Input: part model. Units: mm. Frame: model coordinates. A direction names the side the tool comes from. Coordinates: 2 decimals unless noted, no trailing zeros. Order: outer loops, then holes, each group sorted by start corner. A loop starts at its lowest first (then second) coordinate and runs counter-clockwise, first axis right, second up. Notation, with made-up numbers: (31.5, 54) -> (51.5, 54) arc R22 cw to (51.5, 84) -> close; hole circle Ø10 at (24.25, 70.25). An arc over 180 degrees is marked (long way). One line per question, with ' | ' between items.
```python
from build123d import *

# Parameters (mm, degrees)
F0_W     = 19.05
F0_H     = 19.05
F1_DEPTH = 9.525
F2_R     = 6.35
F3_DEPTH = 12.7
F4_R     = 9.525
F4_R_2   = 6.35
F5_DEPTH = 12.7


with BuildPart() as f1:
    # F0 (on Top) → F1 (new body, symmetric)
    with BuildSketch(Plane.XY):
        Rectangle(F0_W, F0_H)
    extrude(amount=F1_DEPTH, both=True)

    # F2 (on face) → F3 (join)
    with BuildSketch(Plane(origin=(0, 9.525, 0), x_dir=(-1, 0, 0), z_dir=(0, 1, 0))):
        with BuildLine():
            ThreePointArc((0, -9.525), (6.7351920908, -6.7351920908), (9.525, 0))
            ThreePointArc((9.525, 0), (6.7351920908, 6.7351920908), (0, 9.525))
            ThreePointArc((0, 9.525), (-6.7351920908, 6.7351920908), (-9.525, 0))
            ThreePointArc((-9.525, 0), (-6.7351920908, -6.7351920908), (0, -9.525))
        make_face()
        Circle(F2_R, mode=Mode.SUBTRACT)
    extrude(amount=F3_DEPTH)

    # F4 (on face) → F5 (join)
    with BuildSketch(Plane(origin=(-9.525, 0, 0), x_dir=(0, -1, 0), z_dir=(-1, 0, 0))):
        Circle(F4_R)
        Circle(F4_R_2, mode=Mode.SUBTRACT)
    extrude(amount=F5_DEPTH)


solid = f1.part
```
1. Cut plane D-D, the plane y = -5. Return loops of the section in (x, z) (3 decimals).
Recorded:
outline: (-22.225, -8.107) -> (-9.525, -8.107) -> (-9.525, -9.525) -> (9.525, -9.525) -> (9.525, 9.525) -> (-9.525, 9.525) -> (-9.525, 8.107) -> (-22.225, 8.107) -> (-22.225, 3.914) -> (-9.525, 3.914) -> (-9.525, -3.914) -> (-22.225, -3.914) -> close
2. Mould query, pull axis Y, two halves, no side actions, for faces 1 (the face through (-9.525, -8, -7)), 2 (the face through (-15.79, 1.38, -6.2)), 3 (the face through (-6.2, 22.225, -2)), 4 (the face through (-9.525, 0, 0)). Classes: released by +Y, released by -Y, zero draft, split by the parting line, or undercut.
Recorded:
face 1: zero draft | face 2: undercut | face 3: released by +Y | face 4: undercut
3. Cut plane B-B, the plane z = -4. Return loops of the section in (x, y) (3 decimals), and give its area (3 significant figures).
Recorded:
outline: (-22.225, -8.644) -> (-9.525, -8.644) -> (-9.525, -9.525) -> (9.525, -9.525) -> (9.525, 9.525) -> (8.644, 9.525) -> (8.644, 22.225) -> (4.932, 22.225) -> (4.932, 9.525) -> (-4.932, 9.525) -> (-4.932, 22.225) -> (-8.644, 22.225) -> (-8.644, 9.525) -> (-9.525, 9.525) -> (-9.525, 8.644) -> (-22.225, 8.644) -> (-22.225, 4.932) -> (-9.525, 4.932) -> (-9.525, -4.932) -> (-22.225, -4.932) -> close | area: 552 mm^2
4. Access query for faces 5 (the face through (0, 9.525, 0)), 6 (the face through (-15.786, 7.559, -5.796)), 7 (the face through (-8, 9.525, 7)), 8 (the face through (-9.525, 8, -8)), 9 (the face through (8, 9.525, -8)). Directions: +Z, -Z, +X, -X, +Y, -Y. A direction counts if a zero-diameter tool reaches every point of the face in a straight line with its end or side. Return the directions, or none.
Recorded:
face 5: +Y | face 6: -X | face 7: +Z, -X, +Y | face 8: -Z, -X, +Y | face 9: -Z, +X, +Y
5. Cut plane A-A, the plane x = -19. Return loops of the section in (y, z) (3 decimals).
Recorded:
outline: circle Ø19.05 at (0, 0); hole circle Ø12.7 at (0, 0)
6. Ray query, line 1 (Z direction, x = -12, y = 0) (3 decimals); line 2 (Y direction, x = 0, z = -3.5) (3 decimals). Return the intervals inside material, ascending. Write a range as [from, to].
Recorded:
line 1: z = [-9.525, -6.35], [6.35, 9.525] | line 2: y = [-9.525, 9.525]
7. Cut plane C-C, the plane x = -4.5. Return loops of the section in (y, z) (3 decimals), and give its area (3 significant figures).
Recorded:
outline: (-9.525, -9.525) -> (9.525, -9.525) -> (9.525, -8.395) -> (22.225, -8.395) -> (22.225, -4.48) -> (9.525, -4.48) -> (9.525, 4.48) -> (22.225, 4.48) -> (22.225, 8.395) -> (9.525, 8.395) -> (9.525, 9.525) -> (-9.525, 9.525) -> close | area: 462 mm^2
8. Pin query (flat end, axial travel): pin 1 Ø5 at (y, z) = (12.5, -1) entering from -X (3 decimals); pin 2 Ø1 at (y, z) = (17, 7) entering from -X; pin 3 Ø10 at (x, y) = (-12.5, 15.5) entering from +Z. Return the tip coordinate at first contact, or that it passes through.
Recorded:
pin 1: stops at x = -9.525 | pin 2: stops at x = -6.96 | pin 3: stops at z = 5.87
